Check sheet for the modelled part. Datum: model origin and axes. Units: mm. Face numbers are marked on the shaded views. A direction names the side the tool comes from. Give positions to 0.01 mm unless a question says otherwise; leave off trailing zeros. Order: outer loops, then holes, each group sorted by start corner. A loop starts at its lowest first (then second) coordinate and runs counter-clockwise, first axis right, second up.
```python
from build123d import *

# Parameters (mm, degrees)
F0_W     = 82.0065811276
F0_H     = 55.3618445992
F1_DEPTH = 85
F3_DEPTH = 81.9
F4_W     = 70.7565844059
F4_H     = 44.7039492428
F5_DEPTH = 85
F6_W     = 30.9852808714
F6_H     = 6.8782754242
F6_H_2   = 5.6699812412
F6_W_2   = 11.9137810543
F6_H_3   = 24.3619084358
F7_DEPTH = 55
F9_START = -30.5
F8_W     = 55.3618445992
F8_H     = 5.8199772239
F9_DEPTH = 48


with BuildPart() as f1:
    # F0 (on Top) → F1 (new body)
    with BuildSketch(Plane.XY):
        Rectangle(F0_W, F0_H)
    extrude(amount=F1_DEPTH)

    # F2 (on face) → F3 (join)
    with BuildSketch(Plane(origin=(-41.0032905638, 0, 0), x_dir=(0, -1, 0), z_dir=(-1, 0, 0))):
        Polygon((27.6809222996, 0), (-27.6809222996, 0), (0, -15.9815879411), align=None)
    extrude(amount=-F3_DEPTH)

    # F4 (on face) → F5 (cut)
    with BuildSketch(Plane.XY.offset(85)):
        Rectangle(F4_W, F4_H)
    extrude(amount=-F5_DEPTH, mode=Mode.SUBTRACT)

    # F6 (on face) → F7 (cut)
    with BuildSketch(Plane(origin=(-41.0032905638, 0, 0), x_dir=(0, -1, 0), z_dir=(-1, 0, 0))):
        with Locations((0, 14.1018014401)):
            Rectangle(F6_W, F6_H)
        with Locations((0, 34.5212779939)):
            Rectangle(F6_W, F6_H_2)
        with Locations((-0.3322646953, 72.8002712131)):
            Rectangle(F6_W_2, F6_H_3)
    extrude(amount=-F7_DEPTH, mode=Mode.SUBTRACT)

    # F8 (on face) → F9 (join)
    with BuildSketch(Plane.YZ.offset(41.0032905638).offset(F9_START)):
        with Locations((0, 42.5)):
            Rectangle(F8_W, F8_H)
    extrude(amount=-F9_DEPTH)


solid = f1.part
```
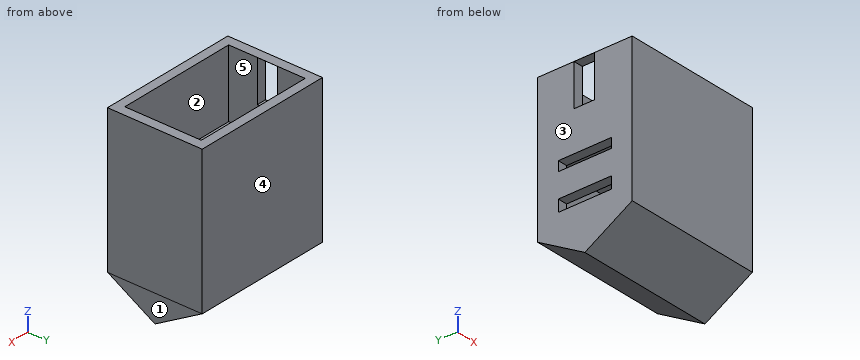
(1) Sectioned sample at B-B (y = -10.5). Enter the section's corners in (x, z), plus the area to 3 significant figures.
(2) Sectioned sample at A-A (x = -18). Enter the section's corners in (y, z).
(3) Go/stop test with flat-tipped pins: P1, Ø8, axis at x = -18, y = 13, coming from the +Z side; P2, Ø6, axis at x = -25.5, y = 8, coming from the -Z side; P3, Ø13, axis at y = -5.5, z = -7.5, coming from the +X side. Record where each tip stops, or that it passes through.
(4) Tool access check on the marked faces 4 and 5. Record the directions out of +Z, -Z, +X, -X, +Y, -Y that give a thin tool (end or side, any length) a straight path to the whole face; none if there is none.
(5) Sectioned sample at D-D (x = 18). Enter the section's corners in (y, z).
(6) Sectioned sample at C-C (z = 52). Enter the section's corners in (x, y).
(7) Release check for a two-part mould opening along X. For the marked faces 1, 2 and 3 record: released by +X, released by -X, zero draft, split by the parting line, or undercut.
(8) Thickness scan on L1, parallel to X at y = -21, z = 72; L2, parallel to Y at x = 15.5, z = 55; L3, parallel to Y at x = -36.5, z = 70.5. Record the ranges inside material, lowest first.
Values follow:
1. outline: (-41, -9.92) - (40.9, -9.92) - (40.9, 0) - (41, 0) - (41, 85) - (35.38, 85) - (35.38, 0) - (-35.38, 0) - (-35.38, 10.66) - (-41, 10.66) - close; (-41, 17.54) - (-35.38, 17.54) - (-35.38, 31.69) - (-41, 31.69) - close; (-41, 37.36) - (-35.38, 37.36) - (-35.38, 39.59) - (10.5, 39.59) - (10.5, 45.41) - (-35.38, 45.41) - (-35.38, 85) - (-41, 85) - close
1. area: 1,970 mm2
2. outline: (-27.68, 0) - (0, -15.98) - (27.68, 0) - (27.68, 85) - (22.35, 85) - (22.35, 45.41) - (-22.35, 45.41) - (-22.35, 85) - (-27.68, 85) - close; hole (-22.35, 0) - (22.35, 0) - (22.35, 39.59) - (-22.35, 39.59) - close
3. P1: stops at z = 45.41
3. P2: stops at z = -13.09
3. P3: stops at x = 40.9
4. face 4: +Z, -Z, +X, -X, +Y
4. face 5: +Z
5. outline: (-27.68, 0) - (0, -15.98) - (27.68, 0) - (27.68, 85) - (22.35, 85) - (22.35, 0) - (-22.35, 0) - (-22.35, 85) - (-27.68, 85) - close
6. outline: (-41, -27.68) - (41, -27.68) - (41, 27.68) - (-41, 27.68) - close; hole (-35.38, -22.35) - (35.38, -22.35) - (35.38, 22.35) - (-35.38, 22.35) - close
7. face 1: released by +X
7. face 2: undercut
7. face 3: released by -X
8. L1: x = -41 to -35.38, 35.38 to 41
8. L2: y = -27.68 to -22.35, 22.35 to 27.68
8. L3: y = -27.68 to -5.62, 6.29 to 27.68
